Input: dimensioned drawing with shaded views. Units: mm. Origin: part minimum x, y, z. Coordinates: 2 decimals unless noted, no trailing zeros. Order: outer loops, then holes, each group sorted by start corner. A loop starts at its lowest first (then second) coordinate and runs counter-clockwise, first axis right, second up.
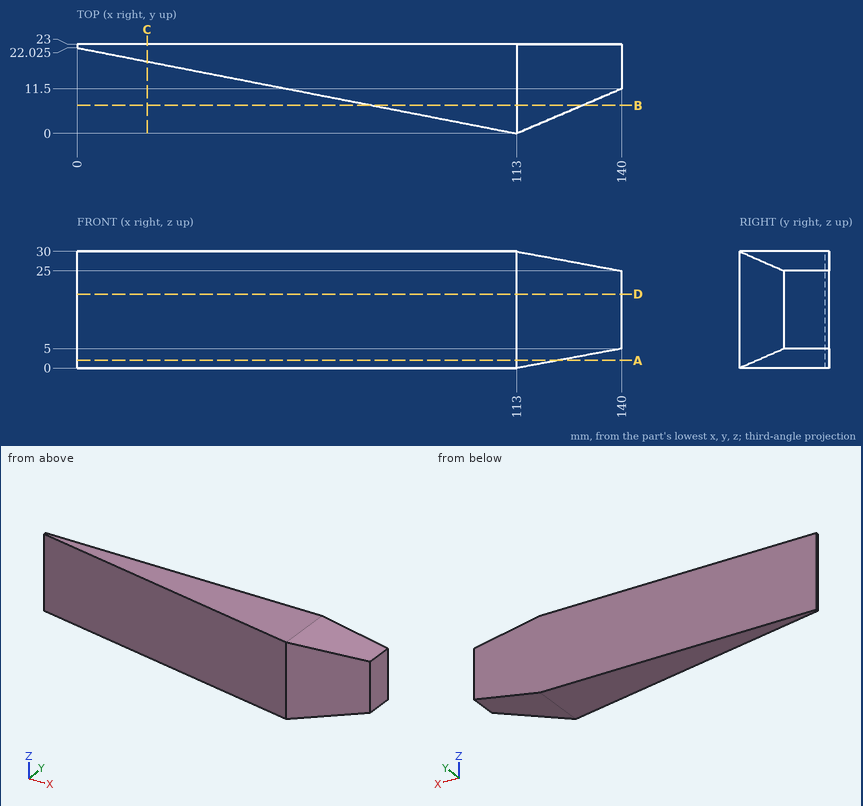
1. Section query A-A on z = 2. Return loops of the section in (x, y) (1 decimal), plus the area to 3 significant figures.
Findings:
outline: (0, 22) - (113, 0) - (123.8, 4.6) - (123.8, 23) - (0, 23) - close
area: 1,580 mm2
2. Pin query (flat end, axial travel): P1, Ø1.5, axis at x = 17, z = 8.5, coming from the -Y side (1 decimal); P2, Ø2, axis at x = 43.5, z = 11, coming from the -Y side; P3, Ø5, axis at y = 2.5, z = 5, coming from the +X side. Return the tip coordinate at first contact, or that it passes through.
Findings:
P1: stops at y = 18.6
P2: stops at y = 13.35
P3: stops at x = 124.74
3. Section query C-C on x = 18. Return loops of the section in (y, z).
Findings:
outline: (18.52, 0) - (23, 0) - (23, 30) - (18.52, 30) - close
4. Ray query, line 1 (Y direction, x = 18, z = 24.5); line 2 (Y direction, x = 103, z = 9); line 3 (Z direction, x = 128, y = 8.75). Return the intervals inside material, ascending.
Findings:
line 1: y = 18.52 to 23
line 2: y = 1.95 to 23
line 3: z = 2.78 to 27.22
5. Section query D-D on z = 19. Return loops of the section in (x, y) (1 decimal), plus the area to 3 significant figures.
Findings:
outline: (0, 22) - (113, 0) - (140, 11.5) - (140, 23) - (0, 23) - close
area: 1,820 mm2
6. Section query B-B on y = 7.25. Return loops of the section in (x, z) (1 decimal), plus the area to 3 significant figures.
Findings:
outline: (75.8, 0) - (113, 0) - (130, 3.2) - (130, 26.8) - (113, 30) - (75.8, 30) - close
area: 1,570 mm2
